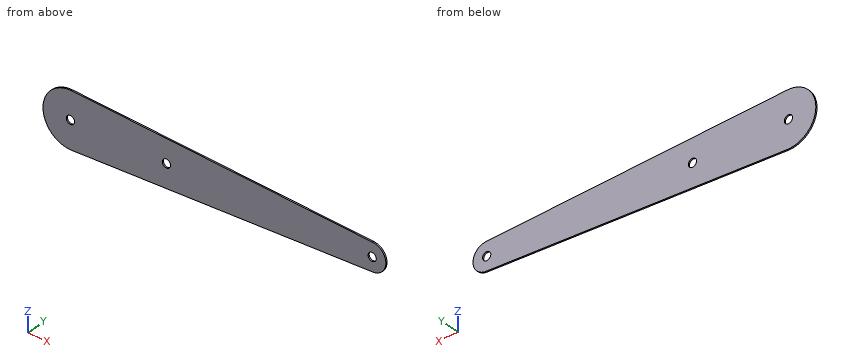
```python
from build123d import *

# Parameters (mm, degrees)
BOSS_EXTRUDE1_DEPTH = 2.54
SKETCH2_R           = 7.5
CUT_EXTRUDE1_DEPTH  = 10


with BuildPart() as part:
    # Sketch1 → Boss-Extrude1 (new body)
    with BuildSketch(Plane(origin=(0, 0, 0), x_dir=(1, 0, 0), z_dir=(0, 1, 0))):
        with BuildLine():
            Line((-247.724918783, 49.948213236), (300, 25))
            ThreePointArc((300, 25), (325, 0), (300, -25))
            Line((300, -25), (-247.724918783, -49.948213236))
            ThreePointArc((-247.724918783, -49.948213236), (-300, 0), (-247.724918783, 49.948213236))
        make_face()
    extrude(amount=BOSS_EXTRUDE1_DEPTH)

    # Sketch2 → Cut-Extrude1 (cut)
    with BuildSketch(Plane(origin=(0, 2.54, 0), x_dir=(1, 0, 0), z_dir=(0, 1, 0))):
        with Locations(Location((-75, 0, 0), (0, 0, 270))):
            Circle(SKETCH2_R)
        with Locations(Location((300, 0, 0), (0, 0, 270))):
            Circle(SKETCH2_R)
        with Locations(Location((-250, 0, 0), (0, 0, 270))):
            Circle(SKETCH2_R)
    extrude(amount=-CUT_EXTRUDE1_DEPTH, mode=Mode.SUBTRACT)


solid = part.part
```
CAD build for the part. Positions are in the model's coordinates, mm. Coordinates: 2 decimals unless noted, no trailing zeros. Order: outer loops, then holes, each group sorted by start corner. A loop starts at its lowest first (then second) coordinate and runs counter-clockwise, first axis right, second up. Notation, with made-up numbers: (-27, -13.75) - (12, -13.75) arc R26 ccw to (12, 3.25) - close; hole circle Ø8 at (59, -1). An arc over 180 degrees is marked (long way). Answer in a Markdown table with one row per item.
1. Slice it at C-C, the plane x = -75. List the corners of the cut face in (y, z), then the cut area to 3 significant figures.
Answer:
| item | result |
|---|---|
| outline | (0, -42.08) - (2.54, -42.08) - (2.54, -7.5) - (0, -7.5) - close; (0, 7.5) - (2.54, 7.5) - (2.54, 42.08) - (0, 42.08) - close |
| area | 176 mm² |
2. Slice it at A-A, the plane z = 0. List the corners of the cut face in (x, y), then the cut area to 3 significant figures.
Answer:
| item | result |
|---|---|
| outline | (-300, 0) - (-257.5, 0) - (-257.5, 2.54) - (-300, 2.54) - close; (-242.5, 0) - (-82.5, 0) - (-82.5, 2.54) - (-242.5, 2.54) - close; (-67.5, 0) - (292.5, 0) - (292.5, 2.54) - (-67.5, 2.54) - close; (307.5, 0) - (325, 0) - (325, 2.54) - (307.5, 2.54) - close |
| area | 1,470 mm² |
3. Slice it at B-B, the plane y = 0.6. List the corners of the cut face in (x, z).
Answer:
| item | result |
|---|---|
| outline | (-247.72, -49.95) - (300, -25) arc R25 ccw to (300, 25) - (-247.72, 49.95) arc R50 ccw (long way) to start; hole circle Ø15 at (-250, 0); hole circle Ø15 at (-75, 0); hole circle Ø15 at (300, 0) |
4. Drill centre lines: L1, parallel to X at y = 1.75, z = -1; L2, parallel to X at y = 2.3, z = -1.5; L3, parallel to Z at x = -48, y = 0.2. Where is each one in solid material? Low to high. Write a range as from..to.
Answer:
| item | result |
|---|---|
| L1 | -299.99..-257.43, -242.57..-82.43, -67.57..292.57, 307.43..324.98 |
| L2 | -299.98..-257.35, -242.65..-82.35, -67.65..292.65, 307.35..324.95 |
| L3 | -40.85..40.85 |
5. Slice it at D-D, the plane z = -33.5. List the corners of the cut face in (x, y).
Answer:
| item | result |
|---|---|
| outline | (-287.12, 0) - (113.39, 0) - (113.39, 2.54) - (-287.12, 2.54) - close |
6. Flat gauge pins, fed straight in: P1, Ø19.5, axis at x = 300, z = 0, coming from the -Y side; P2, Ø1.5, axis at y = 2, z = 22.5, coming from the -X side; P3, Ø1, axis at y = 1.5, z = 17, coming from the +X side. Where does each tip first touch, or does it go through?
Answer:
| item | result |
|---|---|
| P1 | y = 0 |
| P2 | x = -295.02 |
| P3 | x = 318.78 |
